Could you check a few things on this model? Use its own coordinates, in mm. Face numbers are marked on the shaded views. A direction names the side the tool comes from. Round coordinates to 2 decimals unless told otherwise and drop trailing zeros. Loops run counter-clockwise (first coordinate to the right, second up) from the corner with the lowest first, then second, coordinate; pieces in that order, holes last. Notation, with made-up numbers: M 2.25,-19 L 8.25,-19 A9 ccw 8.25,-9 Z; hole C 35,-4.75 d6. An arc over 180 degrees is marked long. One line per item, written item: value. Start each with the question number.
Q1. Which directions (+Z, -Z, +X, -X, +Y, -Y) give clear straight access to the entire face, cutting with the end or side of a thin tool? Please do the marked faces 1 and 2.
Q2. Imagine slicing it at D-D (z = 3.25). Please give me the cut outline in (x, y), then the cut area to 3 significant figures.
Q3. Imagine slicing it at A-A (z = 0). Please give me the cut outline in (x, y), then the cut area to 3 significant figures.
Q4. Please list where these lines run through material, in increasing order: line 1 along Z through (x, y) = (1.75, 2); line 2 along X through (y, z) = (2.7, 0).
Q5. Imagine slicing it at B-B (x = 0). Please give me the cut outline in (y, z), then the cut area to 3 significant figures.
Q6. Imagine slicing it at C-C (y = 0.65). Please give me the cut outline in (x, z), then the cut area to 3 significant figures.
Q7. Thinking about a two-plate mould opening in Z: for the marked faces 3, 4 and 5, which applies, released by +Z, released by -Z, zero draft, split by the parting line, or undercut?
from build123d import *

# Parameters (mm, degrees)
SKETCH1_W           = 8
SKETCH1_H           = 8
SKETCH1_W_2         = 7
SKETCH1_H_2         = 7
BOSS_EXTRUDE1_DEPTH = 2.94
SKETCH2_W           = 8
SKETCH2_H           = 8
SKETCH2_R           = 3
BOSS_EXTRUDE2_DEPTH = 0.5


with BuildPart() as part:
    # Sketch1 → Boss-Extrude1 (new body)
    with BuildSketch(Plane(origin=(0, 0, 0), x_dir=(1, 0, 0), z_dir=(0, 1, 0))):
        Rectangle(SKETCH1_W, SKETCH1_H)
        Rectangle(SKETCH1_W_2, SKETCH1_H_2, mode=Mode.SUBTRACT)
    extrude(amount=BOSS_EXTRUDE1_DEPTH)

    # Sketch2 → Boss-Extrude2 (add)
    with BuildSketch(Plane(origin=(0, 2.94, 0), x_dir=(1, 0, 0), z_dir=(0, 1, 0))):
        Rectangle(SKETCH2_W, SKETCH2_H)
        with Locations(Location((0, 0, 0), (0, 0, 270))):
            Circle(SKETCH2_R, mode=Mode.SUBTRACT)
    extrude(amount=-BOSS_EXTRUDE2_DEPTH)


solid = part.part
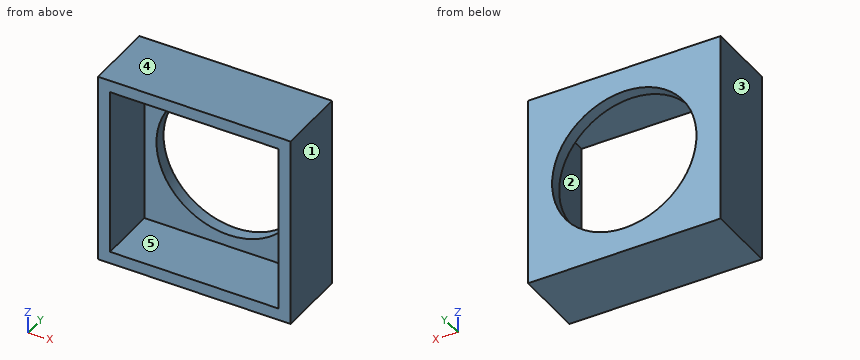
Report:
1. face 1: +Z, -Z, +X, +Y, -Y
1. face 2: -Y
2. outline: M -4,0 L -3.5,0 L -3.5,2.44 L 3.5,2.44 L 3.5,0 L 4,0 L 4,2.94 L -4,2.94 Z
2. area: 6.44 mm²
3. outline: M -4,0 L -3.5,0 L -3.5,2.44 L -3,2.44 L -3,2.94 L -4,2.94 Z; M 3,2.44 L 3.5,2.44 L 3.5,0 L 4,0 L 4,2.94 L 3,2.94 Z
3. area: 3.44 mm²
4. line 1: z = -4 to -3.5, 3.5 to 4
4. line 2: x = -4 to -3, 3 to 4
5. outline: M 0,-4 L 2.94,-4 L 2.94,-3 L 2.44,-3 L 2.44,-3.5 L 0,-3.5 Z; M 0,3.5 L 2.44,3.5 L 2.44,3 L 2.94,3 L 2.94,4 L 0,4 Z
5. area: 3.44 mm²
6. outline: M -4,-4 L 4,-4 L 4,4 L -4,4 Z; hole M -3.5,-3.5 L 3.5,-3.5 L 3.5,3.5 L -3.5,3.5 Z
6. area: 15.0 mm²
7. face 3: zero draft
7. face 4: released by +Z
7. face 5: undercut
